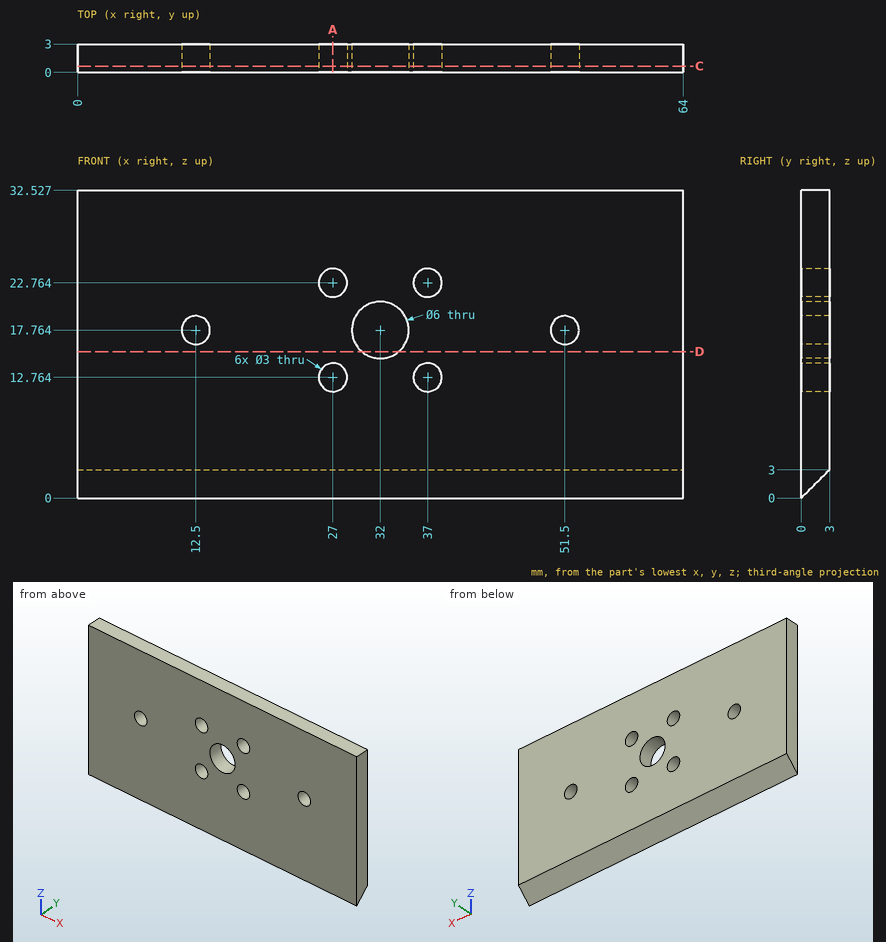
Design review of the part shown in the three views and the two pictorial views. Dimensions are in mm from the part's minimum x, y and z. Round coordinates to 2 decimals unless told otherwise and drop trailing zeros. Loops run counter-clockwise (first coordinate to the right, second up) from the corner with the lowest first, then second, coordinate; pieces in that order, holes last. Notation, with made-up numbers: (-14, -33) - (26, -33) arc R19 ccw to (26, -2) - close; hole circle Ø10 at (-18.75, 61.5). An arc over 180 degrees is marked (long way). One line per item, written item: value. Start each with the question number.
Item 1: Clearance check with flat-ended pins moving along their axes: pin 1 Ø2 at (x, z) = (16, 15) entering from -Y; pin 2 Ø2.5 at (x, z) = (37, 12.76) entering from -Y. State where each tip first meets the part, or that it passes through.
Item 2: Take a section at A-A (x = 27). State how many separate pieces and enclosed holes the cut face has.
Item 3: Take a section at C-C (y = 0.65). Give the boundary of the cut face in (x, z), plus the area to 3 significant figures.
Item 4: For L1, parallel to X at y = 2.5, z = 18; L2, parallel to X at y = 0.3, z = 20; L3, parallel to Z at x = 11.5, y = 1.8 (1 decimal), list the stretches that pass through material, from the lowest coordinate up.
Item 5: Take a section at D-D (z = 15.5). Give the boundary of the cut face in (x, y).
Answer below:
1. pin 1: stops at y = 0
1. pin 2: passes through
2. separate pieces: 3
2. enclosed holes: 0
3. outline: (0, 0.65) - (64, 0.65) - (64, 32.53) - (0, 32.53) - close; hole circle Ø3 at (12.5, 17.76); hole circle Ø3 at (27, 12.76); hole circle Ø3 at (27, 22.76); hole circle Ø6 at (32, 17.76); hole circle Ø3 at (37, 12.76); hole circle Ø3 at (37, 22.76); hole circle Ø3 at (51.5, 17.76)
3. area: 1,970 mm2
4. L1: x = 0 to 11.02, 13.98 to 29.01, 34.99 to 50.02, 52.98 to 64
4. L2: x = 0 to 30, 34 to 64
4. L3: z = 1.8 to 16.6, 18.9 to 32.5
5. outline: (0, 0) - (30.03, 0) - (30.03, 3) - (0, 3) - close; (33.97, 0) - (64, 0) - (64, 3) - (33.97, 3) - close
